```python
from build123d import *

# Parameters (mm, degrees)
F0_W     = 19.05
F0_H     = 19.05
F0_W_2   = 15.875
F0_H_2   = 15.875
F1_DEPTH = 107.95
F2_R     = 1.5875
F3_R     = 1.5875
F4_R     = 3.2385
F4_R_2   = 2.5796875
F5_DEPTH = 19.05
F6_DEPTH = 98.425


with BuildPart() as f1:
    # F0 (on Front) → F1 (new body, symmetric)
    with BuildSketch(Plane.XZ):
        Rectangle(F0_W, F0_H)
        with Locations((-0.0127, 0)):
            Rectangle(F0_W_2, F0_H_2, mode=Mode.SUBTRACT)
    extrude(amount=F1_DEPTH, both=True)

    # F2
    f2_edges = [f1.edges().sort_by_distance(p)[0] for p in [
        (-9.525, 0, 9.525),
        (-9.525, 0, -9.525),
        (9.525, 0, -9.525),
        (9.525, 0, 9.525),
    ]]
    fillet(f2_edges, radius=F2_R)

    # F3
    f3_edges = [f1.edges().sort_by_distance(p)[0] for p in [
        (-7.9502, 0, 7.9375),
        (-7.9502, 0, -7.9375),
        (7.9248, 0, 7.9375),
        (7.9248, 0, -7.9375),
    ]]
    fillet(f3_edges, radius=F3_R)

    # F4 (on face) → F5 (cut)
    with BuildSketch(Plane(origin=(-9.525, 0, 0), x_dir=(0, -1, 0), z_dir=(-1, 0, 0))):
        with Locations((-103.1875, 0)):
            Circle(F4_R)
        with Locations((-31.75, 0)):
            Circle(F4_R_2)
        Circle(F4_R_2)
    extrude(amount=-F5_DEPTH, mode=Mode.SUBTRACT)

    # F6 (cut): a face of the model
    f6_faces = [f1.faces().sort_by_distance(p)[0] for p in [
        (-8.2196076836, -107.95, 0),
    ]]
    extrude(f6_faces, amount=-F6_DEPTH, mode=Mode.SUBTRACT)


solid = f1.part
```
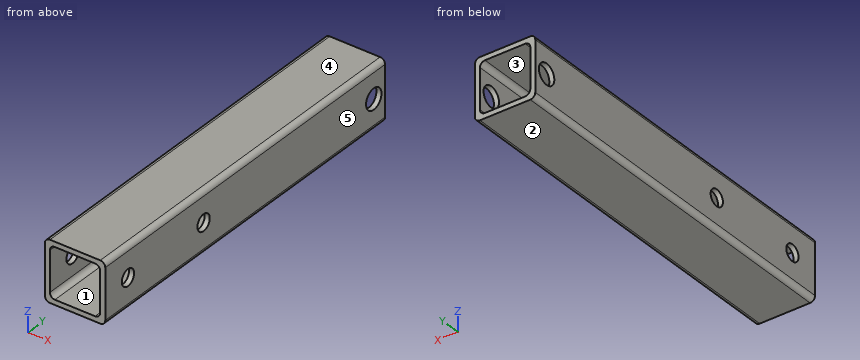
Input: part model. Units: mm. Frame: model coordinates. Face numbers are marked on the shaded views. A direction names the side the tool comes from. Give positions to 0.01 mm unless a question says otherwise; leave off trailing zeros. Use a Markdown table: item, result.
Q1. Pull-direction query (Z, two-part tool) for the marked faces 3, 4 and 5; classes: pulls with the +Z half, pulls with the -Z half, needs draft (parallel to the pull), parting line crosses it, or undercut.
Entries:
| item | result |
|---|---|
| face 3 | undercut |
| face 4 | pulls with the +Z half |
| face 5 | needs draft |
Q2. Ray query, probe 1 along Z at (x, y) = (4, 60) (1 decimal); probe 2 along X at (y, z) = (89.5, -3.25) (3 decimals); probe 3 along X at (y, z) = (4.5, -6.5) (3 decimals). Return the intervals inside material, ascending. Write a range as from..to.
Entries:
| item | result |
|---|---|
| probe 1 | z = -9.5..-7.9, 7.9..9.5 |
| probe 2 | x = -9.525..-7.95, 7.925..9.525 |
| probe 3 | x = -9.525..-7.943, 7.918..9.525 |
Q3. Access query for the marked faces 1 and 2. Directions: +Z, -Z, +X, -X, +Y, -Y. A direction counts if a zero-diameter tool reaches every point of the face in a straight line with its end or side. Return the directions, or none.
Entries:
| item | result |
|---|---|
| face 1 | +Y, -Y |
| face 2 | -Z, +X, -X, +Y, -Y |
Q4. First-contact query: P1, Ø5, axis at x = 7, z = -3, coming from the +Y side. Flat tip, straight axial feed; report the tip coordinate or a pass-through.
Entries:
| item | result |
|---|---|
| P1 | stops at y = 107.95 |
Q5. Section query B-B, the plane z = 0. State how many separate pieces and enclosed holes the cut face has, plus the area to 3 significant figures.
Entries:
| item | result |
|---|---|
| separate pieces | 8 |
| enclosed holes | 0 |
| area | 320 mm² |
